Check sheet for the modelled part. Datum: model origin and axes. Units: mm. A direction names the side the tool comes from. Coordinates: 2 decimals unless noted, no trailing zeros. Write each loop counter-clockwise with the first axis right and the second up, starting at its lowest first coordinate (ties: lowest second). Pieces come first, ordered by that corner, then holes. Notation, with made-up numbers: M 64,-26.75 L 100,-26.75 A24 ccw 100,1.25 Z; hole C 72.5,55.25 d7. An arc over 180 degrees is marked long. Answer as CSV lines item,"result".
from build123d import *

# Parameters (mm, degrees)
SKETCH1_R           = 5
SKETCH1_R_2         = 1.65
BOSS_EXTRUDE1_DEPTH = 5
BOSS_EXTRUDE2_START = 5
BOSS_EXTRUDE2_DEPTH = 5
BOSS_EXTRUDE3_DEPTH = 15
CUT_EXTRUDE1_START  = -1.9
SKETCH4_R           = 2
CUT_EXTRUDE1_DEPTH  = 31.795565449
SKETCH6_R           = 2.75
CUT_EXTRUDE2_DEPTH  = 8
CHAMFER1_SIZE       = 1.2


with BuildPart() as part:
    # Sketch1 → Boss-Extrude1 (new body)
    with BuildSketch(Plane(origin=(0, 0, 0), x_dir=(1, 0, 0), z_dir=(0, 1, 0))):
        with Locations(Location((0, 0, 0), (0, 0, 270))):
            Circle(SKETCH1_R)
        with Locations(Location((0, 0, 0), (0, 0, 270))):
            Circle(SKETCH1_R_2, mode=Mode.SUBTRACT)
    extrude(amount=BOSS_EXTRUDE1_DEPTH)

    # Sketch2 → Boss-Extrude2 (add)
    with BuildSketch(Plane.XZ.offset(BOSS_EXTRUDE2_START)):
        with BuildLine():
            Line((-5, 0), (-5, 30))
            Line((-5, 30), (5, 30))
            Line((5, 30), (5, 0))
            ThreePointArc((5, 0), (0, -5), (-5, 0))
        make_face()
    extrude(amount=-BOSS_EXTRUDE2_DEPTH)

    # Sketch3 → Boss-Extrude3 (add)
    with BuildSketch(Plane.XY.offset(30)):
        with BuildLine():
            Line((-5, 0), (-5, 7))
            ThreePointArc((-5, 7), (0, 2), (5, 7))
            Line((5, 7), (5, 0))
            Line((5, 0), (5, -5))
            Line((5, -5), (-5, -5))
            Line((-5, -5), (-5, 0))
        make_face()
    extrude(amount=-BOSS_EXTRUDE3_DEPTH)

    # Sketch4 → Cut-Extrude1 (cut, through all)
    with BuildSketch(Plane.XZ.offset(5).offset(CUT_EXTRUDE1_START)):
        with Locations(Location((0, 27, 0), (0, 0, 270))):
            Circle(SKETCH4_R)
    extrude(amount=-CUT_EXTRUDE1_DEPTH, mode=Mode.SUBTRACT)

    # Sketch6 → Cut-Extrude2 (cut)
    with BuildSketch(Plane.XZ.offset(5)):
        with Locations(Location((0, 0, 0), (0, 0, 270))):
            Circle(SKETCH6_R)
    extrude(amount=-CUT_EXTRUDE2_DEPTH, mode=Mode.SUBTRACT)

    # Chamfer1
    # the kernel refuses this chamfer: 1.2 mm, written as the material it takes off along each edge
    with BuildSketch(Plane(origin=(0, 3, 0), x_dir=(0, 0, 1), z_dir=(1, 0, 0))) as chamfer1_piece_1_section:
        Polygon((1.65, -CHAMFER1_SIZE), (1.65 + CHAMFER1_SIZE, 0), (1.65, 0), align=None)
    chamfer1_piece_1 = revolve(axis=Axis((0, 3, 0), (0, -1, 0)), mode=Mode.PRIVATE)
    chamfer1_piece_1 = chamfer1_piece_1 & Plane(origin=(0, 3.651745374, 0), x_dir=(0, 0, -1), z_dir=(0, -1, 0)) * Cylinder(2.75, 12, mode=Mode.PRIVATE)
    add(chamfer1_piece_1, mode=Mode.SUBTRACT)


solid = part.part
1) Section check A-A, the plane y = 0.75. Record the boundary of the cut face in (x, z), plus the area to 3 significant figures.
Answer key:
outline,"C 0,0 d10; M -5,15 L 5,15 L 5,30 L -5,30 Z; hole C 0,0 d5.5; hole C 0,27 d4"
area,"192 mm2"
2) Section check D-D, the plane y = -2.25. Record the boundary of the cut face in (x, z), plus the area to 3 significant figures.
Answer key:
outline,"M -5,0 A5 ccw 5,0 L 5,30 L -5,30 Z; hole C 0,0 d5.5; hole C 0,27 d4"
area,"303 mm2"
3) Thickness scan on line 1 along Z through (x, y) = (0, 0.5); line 2 along Z through (x, y) = (0, -0.2); line 3 along X through (y, z) = (-2, 0). Record the ranges inside material, lowest first.
Answer key:
line 1,"z = -5 to -2.75, 2.75 to 5, 15 to 25, 29 to 30"
line 2,"z = -5 to -2.75, 2.75 to 25, 29 to 30"
line 3,"x = -5 to -2.75, 2.75 to 5"
4) Mould release check, pull along X, two halves, no side actions. Record for faces 1 (the face through (5, 0, 19)), 2 (the face through (-1, 4.59, -1.31)), 3 (the face through (0, 0, 9)): pulls with the +X half, pulls with the -X half, needs draft (parallel to the pull), parting line crosses it, or undercut.
Answer key:
face 1,"pulls with the +X half"
face 2,"undercut"
face 3,"needs draft"
5) Depth check by flat-ended pin: P1, Ø1, axis at x = 2, z = 25, coming from the +Y side; P2, Ø1.5, axis at x = -2.5, z = 14, coming from the +Y side; P3, Ø5, axis at x = 0, z = 4.5, coming from the +Y side. Enter the tip coordinate at first touch or a pass-through.
Answer key:
P1,"stops at y = 2.67"
P2,"stops at y = 0"
P3,"stops at y = 5"
6) Section check B-B, the plane x = 0. Record the boundary of the cut face in (y, z).
Answer key:
outline,"M -5,-5 L 5,-5 L 5,-1.65 L 4.2,-1.65 L 3.1,-2.75 L -5,-2.75 Z; M -5,2.75 L 3.1,2.75 L 4.2,1.65 L 5,1.65 L 5,5 L 0,5 L 0,15 L 2,15 L 2,25 L -3.1,25 L -3.1,29 L 2,29 L 2,30 L -5,30 Z"
7) Section check C-C, the plane z = 27. Record the boundary of the cut face in (x, y), plus the area to 3 significant figures.
Answer key:
outline,"M -5,-5 L 5,-5 L 5,7 A5 cw 2,2.42 L 2,-3.1 L -2,-3.1 L -2,2.42 A5 cw -5,7 Z"
area,"59.8 mm2"
8) Tool access check on faces 4 (the face through (0, 0, 29)), 5 (the face through (-2.685, -1.007, 0.596)), 6 (the face through (0, 2, 23)). Record the directions out of +Z, -Z, +X, -X, +Y, -Y that give a thin tool (end or side, any length) a straight path to the whole face; none if there is none.
Answer key:
face 4,"+Y"
face 5,"-Y"
face 6,"+Z, +Y"
